Can you work these out from the model? Positions are in its coordinate system, mm. A direction names the side the tool comes from. Round coordinates to 2 decimals unless told otherwise and drop trailing zeros. Loops run counter-clockwise (first coordinate to the right, second up) from the corner with the lowest first, then second, coordinate; pieces in that order, holes last. Notation, with made-up numbers: M -23,47.25 L 24,47.25 A18 cw 24,70.25 Z; hole C 60.25,-16.5 d5. An arc over 180 degrees is marked long. Use a Markdown table: item, result. Add a question column.
```python
from build123d import *

# Parameters (mm, degrees)
F0_R     = 1.8
F1_DEPTH = 7.25
F3_DEPTH = 1.7
F5_DEPTH = 7.25
F7_DEPTH = 10
F9_DEPTH = 3.5


with BuildPart() as f1:
    # F0 (on Top) → F1 (new body)
    with BuildSketch(Plane.XY):
        with BuildLine():
            Line((14.57509, -8.485134), (-15.42491, -8.485134))
            ThreePointArc((-15.42491, -8.485134), (-18.960444, -9.9496), (-20.42491, -13.485134))
            Line((-20.42491, -13.485134), (-20.42491, -15.485134))
            ThreePointArc((-20.42491, -15.485134), (-18.960444, -19.020668), (-15.42491, -20.485134))
            Line((-15.42491, -20.485134), (14.57509, -20.485134))
            ThreePointArc((14.57509, -20.485134), (18.110624, -19.020668), (19.57509, -15.485134))
            Line((19.57509, -15.485134), (19.57509, -13.485134))
            ThreePointArc((19.57509, -13.485134), (18.110624, -9.9496), (14.57509, -8.485134))
        make_face()
        with Locations((-16.12491, -14.485134)):
            Circle(F0_R, mode=Mode.SUBTRACT)
        with Locations((15.27509, -14.485134)):
            Circle(F0_R, mode=Mode.SUBTRACT)
    extrude(amount=F1_DEPTH)

    # F2 (on face) → F3 (join)
    with BuildSketch(Plane.XY.offset(7.25)):
        with BuildLine():
            Line((-12.42491, -0.485134), (-12.42491, -8.485134))
            ThreePointArc((-12.42491, -8.485134), (-8.910192, -16.970415), (-0.42491, -20.485134))
            ThreePointArc((-0.42491, -20.485134), (8.060371, -16.970415), (11.57509, -8.485134))
            Line((11.57509, -8.485134), (11.57509, -0.485134))
            ThreePointArc((11.57509, -0.485134), (8.060371, 8.000148), (-0.42491, 11.514866))
            ThreePointArc((-0.42491, 11.514866), (-8.910192, 8.000148), (-12.42491, -0.485134))
        make_face()
    extrude(amount=F3_DEPTH)

    # F4 (on face) → F5 (join)
    with BuildSketch(Plane(origin=(0, 0, 7.25), x_dir=(1, 0, 0), z_dir=(0, 0, -1))):
        with BuildLine():
            Line((11.57509, 0.485134), (-12.42491, 0.485134))
            ThreePointArc((-12.42491, 0.485134), (-0.42491, -11.514866), (11.57509, 0.485134))
        make_face()
    extrude(amount=F5_DEPTH)

    # F6 (on face) → F7 (join)
    with BuildSketch(Plane.XY.offset(8.95)):
        with BuildLine():
            Line((11.57509, -8.485134), (-12.42491, -8.485134))
            ThreePointArc((-12.42491, -8.485134), (-0.42491, -20.485134), (11.57509, -8.485134))
        make_face()
    extrude(amount=F7_DEPTH)

    # F8 (on face) → F9 (join)
    with BuildSketch(Plane.XY.offset(18.95)):
        with BuildLine():
            ThreePointArc((-0.394389, 11.517738), (-8.87967, 8.003019), (-12.394389, -0.482262))
            Line((-12.394389, -0.482262), (-12.394389, -8.482262))
            ThreePointArc((-12.394389, -8.482262), (-8.87967, -16.967543), (-0.394389, -20.482262))
            ThreePointArc((-0.394389, -20.482262), (8.090893, -16.967543), (11.605611, -8.482262))
            Line((11.605611, -8.482262), (11.605611, -0.482262))
            ThreePointArc((11.605611, -0.482262), (8.090893, 8.003019), (-0.394389, 11.517738))
        make_face()
    extrude(amount=F9_DEPTH)


solid = f1.part
```
(1) Suppose I cut it at B-B on z = 5.75. List the corners of the cut face in (x, y) for me.
(2) Suppose I cut it at D-D on y = -15. Count the separate pieces of the cut face and the enclosed holes in it, and give its area (3 significant figures).
(3) Suppose I cut it at C-C on x = -16.5. List the corners of the cut face in (y, z) for me, and give its area (3 significant figures).
(4) Thinking about a two-plate mould opening in Y: for faces 6 (the face through (18.07, -19.06, 3.57)), 7 (the face through (11.606, -5, 21)), 8 (the face through (0, -8.485, 4)), which applies, released by +Y, released by -Y, zero draft, split by the parting line, or undercut?
(5) Suppose I cut it at A-A on y = -5. List the corners of the cut face in (x, z) for me, and give its area (3 significant figures).
(6) I'm going to push flat-ended pins straight in: pin 1 (12 mm diameter, centred on x = 13.5, z = 19, fed in from -Y); pin 2 (10 mm diameter, centred on x = 2, z = 9.5, fed in from +Y); pin 3 (4 mm diameter, centred on y = -13.5, z = 18, fed in from +X). Where does each tip first touch, or does it pass through?
(7) If I drill on probe 1 along Z at (x, y) = (-16, -17); probe 2 along Y at (x, z) = (-13, 6.25); probe 3 along Z at (x, y) = (7.5, -2), over which ranges is the centre line in solid material (lowest first)? Write a range as [from, to].
(8) On a 3-axis mill with a long thin cutter (end or side, diameter ignored), from which of +Z, -Z, +X, -X, +Y, -Y can I reach the whole of each face in a straight line? I mean faces 1 (the face through (-18.92, -9.91, 3.57)), 2 (the face through (-1, -4, 7.25)), 3 (the face through (-16.36, -12.7, 3.57)), 4 (the face through (-1, -1, 8.95)), 5 (the face through (-13, -16, 7.25)). Say none if no direction works.
Results below:
| question | item | result |
|---|---|---|
| 1 | outline | M -20.42,-15.49 A5 ccw -15.42,-20.49 L 14.58,-20.49 A5 ccw 19.58,-15.49 L 19.58,-13.49 A5 ccw 14.58,-8.49 L -15.42,-8.49 A5 ccw -20.42,-13.49 Z; M -12.42,-0.49 L 11.58,-0.49 A12 ccw Z; hole C -16.12,-14.49 d3.6; hole C 15.28,-14.49 d3.6 |
| 2 | separate pieces | 3 |
| 2 | enclosed holes | 0 |
| 2 | area | 546 mm² |
| 3 | outline | M -20.37,0 L -16.25,0 L -16.25,7.25 L -20.37,7.25 Z; M -12.72,0 L -8.6,0 L -8.6,7.25 L -12.72,7.25 Z |
| 3 | area | 59.8 mm² |
| 4 | face 6 | released by -Y |
| 4 | face 7 | zero draft |
| 4 | face 8 | undercut |
| 5 | outline | M -12.42,7.25 L 11.58,7.25 L 11.58,8.95 L -12.42,8.95 Z; M -12.39,18.95 L 11.61,18.95 L 11.61,22.45 L -12.39,22.45 Z |
| 5 | area | 125 mm² |
| 6 | pin 1 | stops at y = -17.52 |
| 6 | pin 2 | stops at y = 11.51 |
| 6 | pin 3 | stops at x = 11.19 |
| 7 | probe 1 | z = [0, 7.25] |
| 7 | probe 2 | y = [-20.49, -8.49] |
| 7 | probe 3 | z = [7.25, 8.95], [18.95, 22.45] |
| 8 | face 1 | +Z, -Z, -X, +Y |
| 8 | face 2 | -Z, +X, -X |
| 8 | face 3 | +Z, -Z |
| 8 | face 4 | +X, -X, +Y |
| 8 | face 5 | +Z, -X, -Y |
